```python
from build123d import *

# Parameters (mm, degrees)
SKETCH2_R           = 1.7999999999999927
SKETCH2_R_2         = 1.8000000000000014
SKETCH2_R_3         = 1.7999999999999936
SKETCH2_R_4         = 1.8000000000000005
BOSS_EXTRUDE1_DEPTH = 10
CUT_EXTRUDE1_DEPTH  = 86.30841107417254
FILLET1_R           = 3


with BuildPart() as part:
    # Sketch2 → Boss-Extrude1 (new body)
    with BuildSketch(Plane.XY):
        with BuildLine():
            ThreePointArc((-60.998373193608856, 25.417629235091972), (-69.50179079881426, 24.76016426994454), (-65.04884175350759, 17.486127155053257))
            Line((-65.04884175350759, 17.486127155053268), (-65.05000000000001, -37.513872834627236))
            ThreePointArc((-65.05000000000001, -37.513872834627236), (-69.52213595499958, -44.74994081212703), (-61.050000000000004, -45.51387283462723))
            ThreePointArc((-61.05, -45.51387283462723), (-55.75009387067255, -47.34194119111691), (-52.0844733465611, -43.09999999999998))
            Line((-52.084473346561104, -43.09999999999998), (-36.9, -43.09999999999998))
            Line((-36.9, -43.09999999999998), (36.9, -43.09999999999998))
            Line((36.9, -43.09999999999998), (52.07029117317087, -43.09999999999998))
            ThreePointArc((52.07029117317087, -43.09999999999998), (55.68413677612224, -47.459825116743666), (61.04999999999999, -45.65000000000001))
            ThreePointArc((61.04999999999999, -45.65000000000001), (69.52213595499958, -44.8860679774998), (65.04999999999998, -37.650000000000006))
            Line((65.04999999999998, -37.650000000000006), (65.05, 17.349999999999987))
            ThreePointArc((65.05, 17.349999999999984), (69.52213595499958, 24.586067977499784), (61.04999999999999, 25.349999999999994))
            ThreePointArc((61.04999999999999, 25.349999999999994), (57.09985568418244, 27.349751434896987), (53.110619235405444, 25.42916858771037))
            Line((53.110619235405444, 25.42916858771037), (40.839380764594566, 35.020831412289596))
            ThreePointArc((40.839380764594566, 35.020831412289596), (38.528357481793726, 42.827414929058605), (31.900000000000006, 38.09999999999998))
            Line((31.900000000000006, 38.09999999999998), (-31.89999999999999, 38.09999999999998))
            ThreePointArc((-31.899999999999988, 38.09999999999998), (-38.52835748179412, 42.82741492905847), (-40.839380764594004, 35.02083141228891))
            Line((-40.83938076459401, 35.02083141228891), (-53.11061923540529, 25.4291685877102))
            ThreePointArc((-53.11061923540529, 25.4291685877102), (-57.05731471869626, 27.349994649486177), (-60.99837319360884, 25.41762923509198))
        make_face()
        with Locations((-65.05000000000001, -42.513872834627236)):
            Circle(SKETCH2_R, mode=Mode.SUBTRACT)
        with Locations((-57.050000000000004, -42.513872834627236)):
            Circle(SKETCH2_R_2, mode=Mode.SUBTRACT)
        with Locations((-36.9, -38.09999999999998)):
            Circle(SKETCH2_R_2, mode=Mode.SUBTRACT)
        with Locations((36.9, -38.09999999999998)):
            Circle(SKETCH2_R_2, mode=Mode.SUBTRACT)
        with Locations((57.050000000000004, -42.650000000000006)):
            Circle(SKETCH2_R_2, mode=Mode.SUBTRACT)
        with Locations((65.05, -42.650000000000006)):
            Circle(SKETCH2_R, mode=Mode.SUBTRACT)
        with Locations((-65.04884175350765, 22.486127155053268)):
            Circle(SKETCH2_R_3, mode=Mode.SUBTRACT)
        with Locations((-57.050000000000004, 22.349999999999977)):
            Circle(SKETCH2_R_3, mode=Mode.SUBTRACT)
        with Locations((-36.89999999999999, 38.09999999999998)):
            Circle(SKETCH2_R_2, mode=Mode.SUBTRACT)
        with Locations((57.050000000000004, 22.349999999999987)):
            Circle(SKETCH2_R_4, mode=Mode.SUBTRACT)
        with Locations((65.05, 22.34999999999999)):
            Circle(SKETCH2_R_3, mode=Mode.SUBTRACT)
        with Locations((36.900000000000006, 38.09999999999998)):
            Circle(SKETCH2_R_2, mode=Mode.SUBTRACT)
    extrude(amount=BOSS_EXTRUDE1_DEPTH)

    # Sketch3 → Cut-Extrude1 (cut, through all)
    with BuildSketch(Plane.XY.offset(10)):
        with BuildLine():
            Line((-35.941987653909244, 29.964173484996504), (-55.04889348556858, 15.02949522948242))
            Line((-55.04889348556858, 15.02949522948242), (-55.04991738847525, -33.591122423586484))
            Line((-55.04991738847525, -33.591122423586484), (-40.85853798780756, -33.591122423586484))
            ThreePointArc((-40.85853798780756, -33.591122423586484), (-38.65263543886247, -32.3616841304749), (-36.13624745721949, -32.148808350137216))
            Line((-36.13624745721949, -32.148808350137216), (-5.96078383225156, -0.9920288349264463))
            Line((-5.960783832251558, -0.9920288349264474), (-35.941987653909244, 29.964173484996504))
        make_face()
        with BuildLine():
            ThreePointArc((36.13624745721953, -32.148808350137216), (38.65263543886248, -32.36168413047491), (40.85853798780755, -33.591122423586484))
            Line((40.85853798780755, -33.591122423586484), (55.05, -33.591122423586484))
            Line((55.05, -33.591122423586484), (55.05, 15.028630336068145))
            Line((55.05, 15.028630336068145), (35.94198765390981, 29.964173484997207))
            Line((35.94198765390981, 29.964173484997207), (5.960783832251529, -0.9920288349263657))
            Line((5.960783832251532, -0.9920288349263677), (36.13624745721953, -32.148808350137216))
        make_face()
        Polygon((2.842e-14, 5.162601626016247), (27.05748031496067, 33.09999999999998), (-27.05748031496062, 33.09999999999998), align=None)
        Polygon((-5.551e-14, -7.146659295869048), (-25.611566651253955, -33.591122423586484), (25.61156665125385, -33.591122423586484), align=None)
    extrude(amount=-CUT_EXTRUDE1_DEPTH, mode=Mode.SUBTRACT)

    # Fillet1
    fillet1_edges = [part.edges().sort_by_distance(p)[0] for p in [
        (21.04851564473553, -16.57041859253179, 0),
        (20.95138574308067, 14.486072325035423, 0),
        (45.4959938269549, 22.496401910532676, 10),
        (55.05, -9.281246043759168, 10),
        (47.954268993903774, -33.591122423586484, 0),
        (45.49599382695491, 22.49640191053268, -8.9e-16),
        (47.954268993903774, -33.591122423586484, 10),
        (20.95138574308067, 14.48607232503542, 10),
        (21.04851564473553, -16.570418592531794, 10),
        (2.842e-14, 33.09999999999998, 10),
        (-27.05748031496062, 33.09999999999998, 5),
        (13.52874015748035, 19.131300813008114, 10),
        (27.057480314960674, 33.09999999999998, 5),
        (-13.528740157480296, 19.131300813008114, -8.9e-16),
        (2.842e-14, 5.162601626016247, 5),
        (2.842e-14, 33.09999999999998, 0),
        (13.52874015748035, 19.131300813008114, 0),
        (-13.528740157480296, 19.131300813008114, 10),
        (12.805783325626894, -20.368890859727767, 10),
        (-5.551e-14, -7.146659295869048, 5),
        (-5.329e-14, -33.591122423586484, 0),
        (25.611566651253845, -33.591122423586484, 5),
        (-12.805783325627004, -20.368890859727763, -8.9e-16),
        (-25.611566651253955, -33.591122423586484, 5),
        (12.805783325626894, -20.368890859727767, 0),
        (-12.805783325627004, -20.368890859727763, 10),
        (-5.329e-14, -33.591122423586484, 10),
        (-47.9542276881414, -33.591122423586484, 0),
        (-55.04940543702191, -9.280813597052033, 0),
        (-45.49544056973891, 22.49683435723946, 10),
        (-20.9513857430804, 14.486072325035028, 10),
        (-21.048515644735524, -16.57041859253183, 10),
        (-45.49544056973892, 22.496834357239464, 0),
        (-20.9513857430804, 14.48607232503503, 0),
        (-21.04851564473552, -16.57041859253183, 0),
        (-55.04940543702192, -9.280813597052033, 10),
        (-47.9542276881414, -33.591122423586484, 10),
        (65.04999999999998, -10.15000000000001, 10),
    ]]
    fillet(fillet1_edges, radius=FILLET1_R)


solid = part.part
```
Source: CAD feature listing. Evaluate the final solid. Frame: model axes, mm. A direction names the side the tool comes from. Coordinates: 2 decimals unless noted, no trailing zeros. One line per item, written item: value.
1) Cut plane A-A on x = 0. State how many separate pieces and enclosed holes the cut face has, plus the area to 3 significant figures.
Computed values:
separate pieces: 3
enclosed holes: 0
area: 279 mm^2
2) Reachability of faces 1 (the face through (48.05, -34.49, 0.86)), 2 (the face through (-45.362, 22.601, 5.028)), 3 (the face through (-12.198, -18.444, 9.145)) from +Z, -Z, +X, -X, +Y, -Y: full face, straight path, thin tool, end or side. Return the list, or none.
Computed values:
face 1: -Z
face 2: +Z, -Z
face 3: +Z
3) Ray query, line 1 (X direction, y = -42.65, z = 4.5); line 2 (X direction, y = 13, z = 0.75); line 3 (Y direction, x = -57.05, z = 7). Return the intervals inside material, ascending. Write a range as [from, to].
Computed values:
line 1: x = [-70.05, -66.84], [-63.26, -58.84], [-55.26, 55.25], [58.85, 63.25], [66.85, 70.05]
line 2: x = [-65.05, -56.06], [-18.1, -9], [9, 18.1], [55.05, 65.05]
line 3: y = [-47.51, -44.31], [-40.71, 20.55], [24.15, 27.35]
4) Contact query for flat-ended pins moving along their axis: pin 1 (4.5 mm diameter, centred on x = 46, z = 6, fed in from +Y); pin 2 (4 mm diameter, centred on y = -4, z = 7.5, fed in from -X); pin 3 (2 mm diameter, centred on x = 17, z = 3, fed in from -Y); pin 4 (4 mm diameter, centred on x = 57.05, y = -42.65, fed in from -Z). Output: stop coordinate, or through.
Computed values:
pin 1: stops at y = 32.75
pin 2: stops at x = -65.05
pin 3: stops at y = -43.1
pin 4: stops at z = 0
